Verification items for this drawing (mm, ordinates from the low corner). A direction names the side the tool comes from. Give positions to 0.01 mm unless a question says otherwise; leave off trailing zeros. Loops run counter-clockwise (first coordinate to the right, second up) from the corner with the lowest first, then second, coordinate; pieces in that order, holes last. Notation, with made-up numbers: (5.25, 79.5) -> (45.25, 79.5) arc R6 cw to (45.25, 87.5) -> close; hole circle Ø8 at (11, 40). An arc over 180 degrees is marked (long way). Write item = value, one per line.
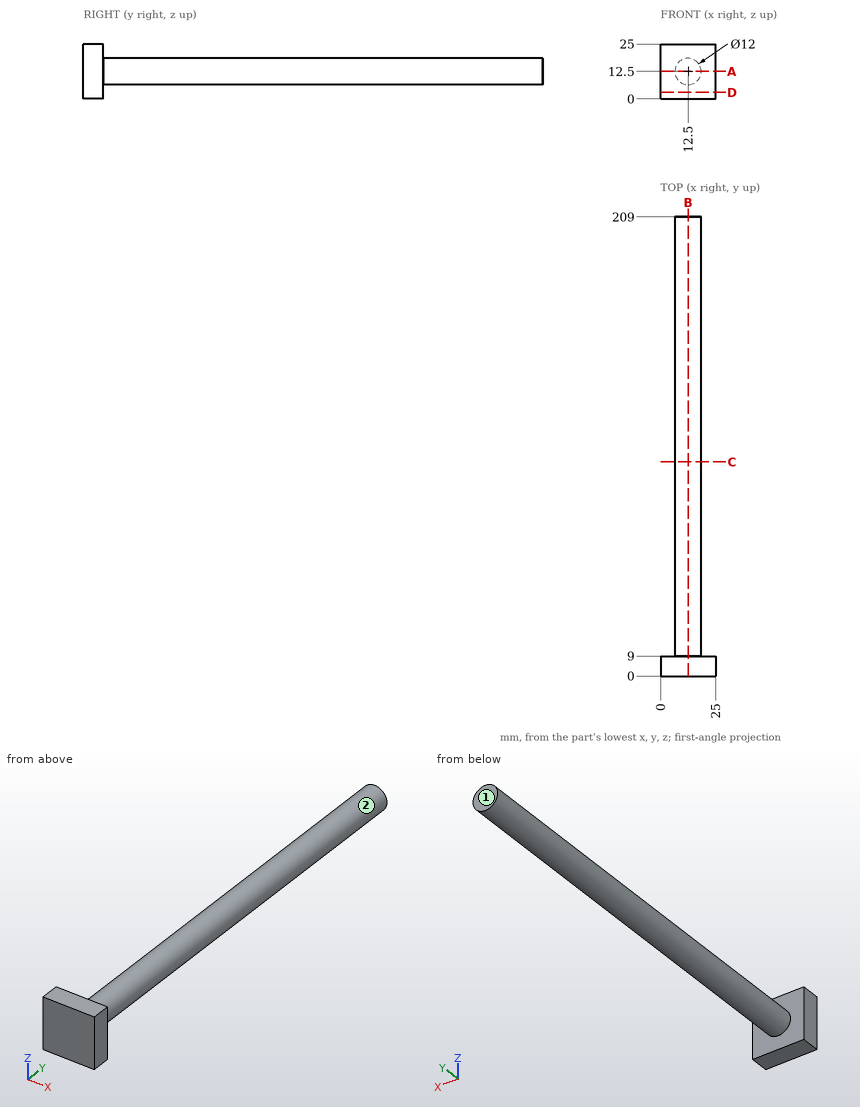
Item 1: Section check C-C, the plane y = 97.5. Record the cut outline in (x, z), plus the area to 3 significant figures.
Answer:
outline = circle Ø12 at (12.5, 12.5)
area = 113 mm^2
Item 2: Tool access check on the marked faces 1 and 2. Record the directions out of +Z, -Z, +X, -X, +Y, -Y that give a thin tool (end or side, any length) a straight path to the whole face; none if there is none.
Answer:
face_1 = +Z, -Z, +X, -X, +Y
face_2 = +Y
Item 3: Section check A-A, the plane z = 12.5. Record the cut outline in (x, y).
Answer:
outline = (0, 0) -> (25, 0) -> (25, 9) -> (18.5, 9) -> (18.5, 209) -> (6.5, 209) -> (6.5, 9) -> (0, 9) -> close
Item 4: Gauge pin test, flat ends, axial feed: pin 1 (10 mm diameter, centred on y = 117.5, z = 11, fed in from +X); pin 2 (6 mm diameter, centred on x = 15.5, y = 132.5, fed in from +Z); pin 3 (6 mm diameter, centred on y = 54.5, z = 8.5, fed in from -X). Record the tip position at first contact, or that the pin passes through.
Answer:
pin_1 = 18.5
pin_2 = 18.5
pin_3 = 6.58
Item 5: Thickness scan on L1, parallel to Z at x = 12.25, y = 11.5; L2, parallel to Y at x = 4.25, z = 4.75; L3, parallel to X at y = 21, z = 17.75. Record the ranges inside material, lowest first. Write a range as [from, to].
Answer:
L1 = [6.51, 18.49]
L2 = [0, 9]
L3 = [9.6, 15.4]
Item 6: Section check D-D, the plane z = 3. Record the cut outline in (x, y).
Answer:
outline = (0, 0) -> (25, 0) -> (25, 9) -> (0, 9) -> close
Item 7: Section check B-B, the plane x = 12.5. Record the cut outline in (y, z).
Answer:
outline = (0, 0) -> (9, 0) -> (9, 6.5) -> (209, 6.5) -> (209, 18.5) -> (9, 18.5) -> (9, 25) -> (0, 25) -> close
